Verification items for this drawing (mm, ordinates from the low corner). Round coordinates to 2 decimals unless told otherwise and drop trailing zeros. Write each loop counter-clockwise with the first axis right and the second up, starting at its lowest first coordinate (ties: lowest second). Pieces come first, ordered by that corner, then holes. Notation, with made-up numbers: (83, 11.25) - (127, 11.25) arc R11 cw to (127, 32.25) - close; hole circle Ø6 at (32.5, 67). An arc over 180 degrees is marked (long way). One line per question, with ' | ' between items. Start each with the question number.
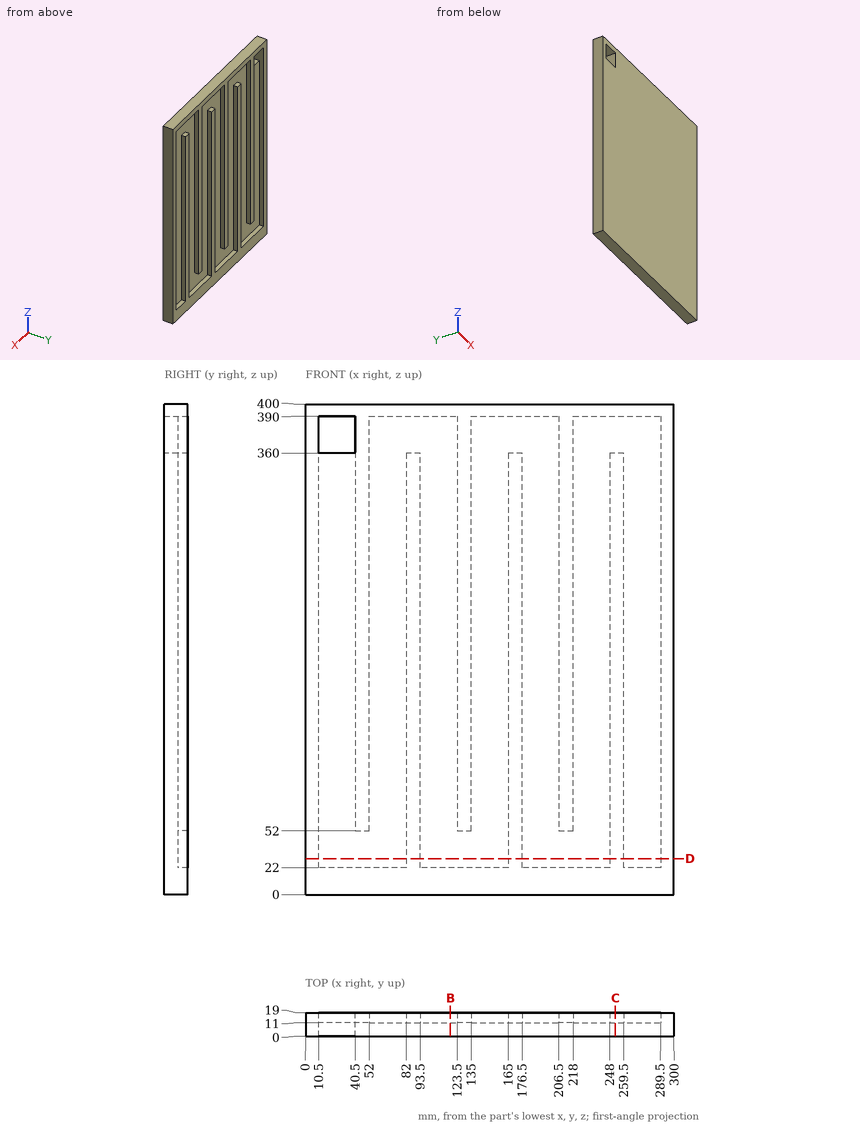
Q1. Go/stop test with a flat-tipped pin: P1, Ø5, axis at x = 74.5, z = 300.5, coming from the +Y side. Record where the tip stops, or that it passes through.
Q2. Section check D-D, the plane z = 29.5. Record the cut outline in (x, y).
Q3. Section check C-C, the plane x = 252.5. Record the cut outline in (y, z).
Q4. Thickness scan on line 1 (X direction, y = 13.25, z = 364); line 2 (Z direction, x = 147.5, y = 14.25); line 3 (X direction, y = 6.75, z = 381.5). Record the ranges inside material, lowest first.
Q5. Section check B-B, the plane x = 118. Record the cut outline in (y, z).
Result sheet:
1) P1: y = 11
2) outline: (0, 0) - (300, 0) - (300, 19) - (289.5, 19) - (289.5, 11) - (259.5, 11) - (259.5, 19) - (248, 19) - (248, 11) - (176.5, 11) - (176.5, 19) - (165, 19) - (165, 11) - (93.5, 11) - (93.5, 19) - (82, 19) - (82, 11) - (10.5, 11) - (10.5, 19) - (0, 19) - close
3) outline: (0, 0) - (19, 0) - (19, 360) - (11, 360) - (11, 390) - (19, 390) - (19, 400) - (0, 400) - close
4) line 1: 0 to 10.5, 40.5 to 52, 123.5 to 135, 206.5 to 218, 289.5 to 300 | line 2: 0 to 22, 390 to 400 | line 3: 0 to 10.5, 40.5 to 300
5) outline: (0, 0) - (19, 0) - (19, 22) - (11, 22) - (11, 390) - (19, 390) - (19, 400) - (0, 400) - close
